The figure shows three views and two pictorial views of one solid part (mm, origin at its lowest corner). Answer the questions. Give positions to 0.01 mm unless a question says otherwise; leave off trailing zeros. Write each loop counter-clockwise with the first axis right and the second up, starting at its lowest first coordinate (ties: lowest second). Pieces come first, ordered by that corner, then holes. Notation, with made-up numbers: (18, -31) - (31, -31) arc R33 cw to (31, -3) - close; hole circle Ø9 at (40, 58). An arc over 180 degrees is marked (long way). One line per question, with ' | ' between items. Start each with the question number.
1. Find the intervals of material crossed by L1, parallel to X at y = 2.5, z = 58.3; L2, parallel to X at y = 1.95, z = 2.5; L3, parallel to Z at x = 37, y = 2.55, in increasing order. Write a range as from..to.
2. A cutting plane is placed at D-D (x = 20). Determine the outline of the cut face in (y, z), then the cut area to 4 significant figures.
3. A cutting plane is placed at C-C (x = 27.5). Determine the outline of the cut face in (y, z).
4. The mould has two halves that part along Z. Classify the marked faces 1 and 2: +Z half, -Z half, draft (parallel to the pull), parting line (faces both ways), or undercut.
5. A cutting plane is placed at B-B (y = 3.2). Determine the outline of the cut face in (x, z), then the cut area to 3 significant figures.
6. A cutting plane is placed at A-A (z = 2.5). Determine the outline of the cut face in (x, y), then the cut area to 4 significant figures.
7. Given P1, Ø3.5, axis at x = 22.5, z = 15.5, coming from the +Y side, flat-ended and moving along its own axis, determine where the tip first touches the part or whether it passes through.
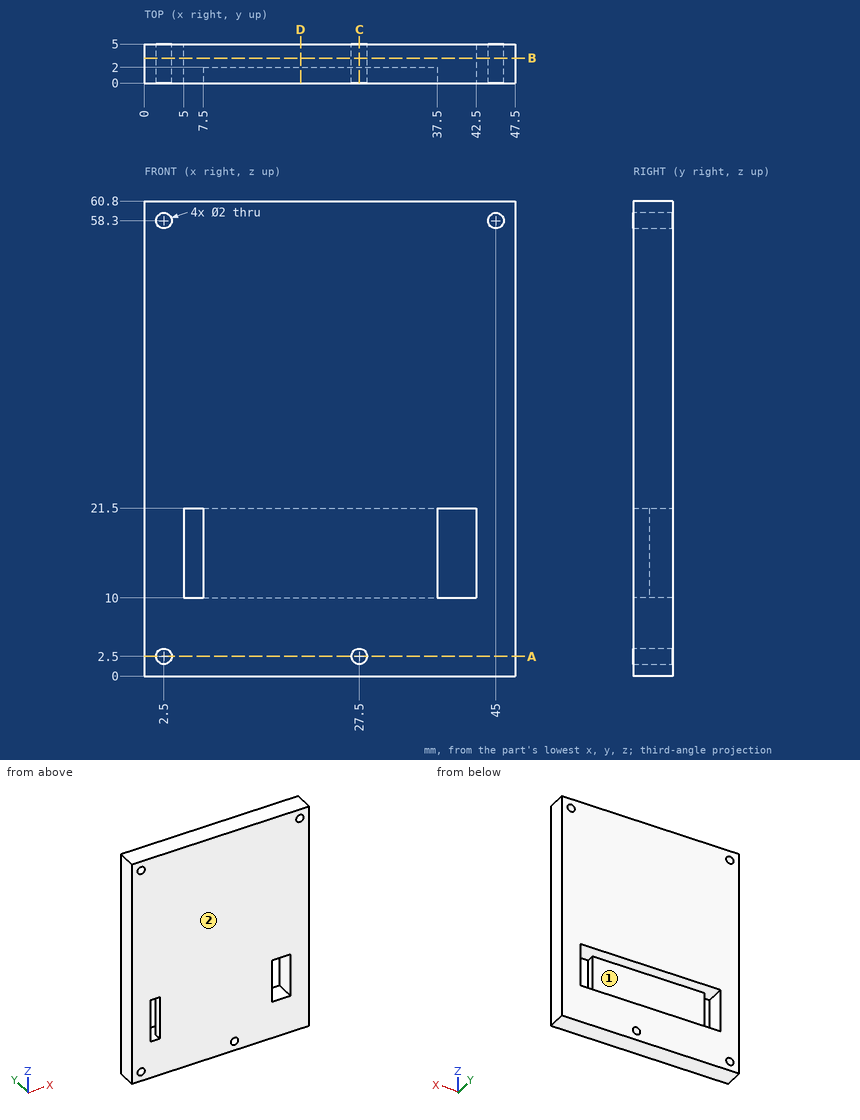
Determined:
1) L1: 0..1.5, 3.5..44, 46..47.5 | L2: 0..1.5, 3.5..26.5, 28.5..47.5 | L3: 0..10, 21.5..60.8
2) outline: (0, 0) - (5, 0) - (5, 10) - (2, 10) - (2, 21.5) - (5, 21.5) - (5, 60.8) - (0, 60.8) - close | area: 269.5 mm2
3) outline: (0, 0) - (5, 0) - (5, 1.5) - (0, 1.5) - close; (0, 3.5) - (5, 3.5) - (5, 10) - (2, 10) - (2, 21.5) - (5, 21.5) - (5, 60.8) - (0, 60.8) - close
4) face 1: undercut | face 2: draft
5) outline: (0, 0) - (47.5, 0) - (47.5, 60.8) - (0, 60.8) - close; hole circle Ø2 at (2.5, 2.5); hole circle Ø2 at (2.5, 58.3); hole (5, 10) - (42.5, 10) - (42.5, 21.5) - (5, 21.5) - close; hole circle Ø2 at (27.5, 2.5); hole circle Ø2 at (45, 58.3) | area: 2,440 mm2
6) outline: (0, 0) - (1.5, 0) - (1.5, 5) - (0, 5) - close; (3.5, 0) - (26.5, 0) - (26.5, 5) - (3.5, 5) - close; (28.5, 0) - (47.5, 0) - (47.5, 5) - (28.5, 5) - close | area: 217.5 mm2
7) P1: y = 2
